from build123d import *

# Parameters (mm, degrees)
SKETCH1_W           = 137.287
SKETCH1_H           = 77.47
BOSS_EXTRUDE1_DEPTH = 17.78
SKETCH2_W           = 132.207
SKETCH2_H           = 67.31
CUT_EXTRUDE1_DEPTH  = 12.7
SKETCH4_R           = 11.43
CUT_EXTRUDE2_DEPTH  = 80.834956737
SKETCH5_W           = 137.287
SKETCH5_H           = 12.7
BOSS_EXTRUDE2_DEPTH = 1.27
SKETCH6_W           = 8.314266468
SKETCH6_H           = 19.05
CUT_EXTRUDE3_DEPTH  = 81.798878193
SKETCH9_W           = 137.287
SKETCH9_H           = 2
SKETCH9_W_2         = 10
SKETCH9_H_2         = 3
BOSS_EXTRUDE4_DEPTH = 3
SKETCH10_R          = 1.44
CUT_EXTRUDE4_DEPTH  = 84.591762855


with BuildPart() as part:
    # Sketch1 → Boss-Extrude1 (new body)
    with BuildSketch(Plane(origin=(0, 0, 0), x_dir=(1, 0, 0), z_dir=(0, 1, 0))):
        Rectangle(SKETCH1_W, SKETCH1_H)
    extrude(amount=BOSS_EXTRUDE1_DEPTH)

    # Sketch2 → Cut-Extrude1 (cut)
    with BuildSketch(Plane(origin=(0, 17.78, 0), x_dir=(1, 0, 0), z_dir=(0, 1, 0))):
        with Locations((2.54, 0)):
            Rectangle(SKETCH2_W, SKETCH2_H)
    extrude(amount=-CUT_EXTRUDE1_DEPTH, mode=Mode.SUBTRACT)

    # Sketch4 → Cut-Extrude2 (cut, through all)
    with BuildSketch(Plane(origin=(0, 5.08, 0), x_dir=(1, 0, 0), z_dir=(0, 1, 0))):
        with Locations(Location((43.7769, 0, 0), (0, 0, 270))):
            Circle(SKETCH4_R)
    extrude(amount=-CUT_EXTRUDE2_DEPTH, mode=Mode.SUBTRACT)

    # Sketch5 → Boss-Extrude2 (add)
    with BuildSketch(Plane(origin=(0, 17.78, 0), x_dir=(1, 0, 0), z_dir=(0, 1, 0))):
        with Locations((0, 32.385)):
            Rectangle(SKETCH5_W, SKETCH5_H)
        with Locations((0, -32.385)):
            Rectangle(SKETCH5_W, SKETCH5_H)
    extrude(amount=BOSS_EXTRUDE2_DEPTH)

    # Sketch6 → Cut-Extrude3 (cut, through all)
    with BuildSketch(Plane(origin=(0, 17.78, 0), x_dir=(1, 0, 0), z_dir=(0, 1, 0))):
        with Locations((-64.486366766, 0)):
            Rectangle(SKETCH6_W, SKETCH6_H)
    extrude(amount=-CUT_EXTRUDE3_DEPTH, mode=Mode.SUBTRACT)

    # Sketch9 → Boss-Extrude4 (add)
    with BuildSketch(Plane(origin=(0, 0, 0), x_dir=(-1, 0, 0), z_dir=(0, -1, 0))):
        with Locations((0, -39.735)):
            Rectangle(SKETCH9_W, SKETCH9_H)
        with Locations((0, 39.735)):
            Rectangle(SKETCH9_W, SKETCH9_H)
        with Locations((53.6435, -42.235)):
            Rectangle(SKETCH9_W_2, SKETCH9_H_2)
        with Locations((53.6435, 42.235)):
            Rectangle(SKETCH9_W_2, SKETCH9_H_2)
        with Locations((33.6435, -42.235)):
            Rectangle(SKETCH9_W_2, SKETCH9_H_2)
        with Locations((33.6435, 42.235)):
            Rectangle(SKETCH9_W_2, SKETCH9_H_2)
    extrude(amount=-BOSS_EXTRUDE4_DEPTH)

    # Sketch10 → Cut-Extrude4 (cut, through all)
    with BuildSketch(Plane(origin=(0, 0, 0), x_dir=(-1, 0, 0), z_dir=(0, -1, 0))):
        with Locations(Location((33.6435, -41.295, 0), (0, 0, 90))):
            Circle(SKETCH10_R)
        with Locations(Location((53.6435, -41.295, 0), (0, 0, 90))):
            Circle(SKETCH10_R)
        with Locations(Location((53.6435, 41.295, 0), (0, 0, 90))):
            Circle(SKETCH10_R)
        with Locations(Location((33.6435, 41.295, 0), (0, 0, 90))):
            Circle(SKETCH10_R)
    extrude(amount=-CUT_EXTRUDE4_DEPTH, mode=Mode.SUBTRACT)


solid = part.part
Source: CAD feature listing. Evaluate the final solid. Frame: model axes, mm. A direction names the side the tool comes from. Give positions to 0.01 mm unless a question says otherwise; leave off trailing zeros. Write each loop counter-clockwise with the first axis right and the second up, starting at its lowest first coordinate (ties: lowest second). Pieces come first, ordered by that corner, then holes. Notation, with made-up numbers: M -21.75,13 L 17.25,13 A7 cw 17.25,22 Z; hole C 29,82 d9. An arc over 180 degrees is marked long. Return JSON: item names as keys, results as strings. Group by question number.
1) Set-up query: faces 4 (the face through (-64, 1, -40.735)), 5 (the face through (21, 1, -40.735)), 6 (the face through (21, 1, 40.735)), 7 (the face through (-65, 9, 9.525)), 8 (the face through (-44, 1, 40.735)). Return all of +Z, -Z, +X, -X, +Y, -Y with unobstructed straight access to the full face (end or side cutting, diameter ignored); none if empty.
2) Pin query (flat end, axial travel): P1, Ø4, axis at y = 8.5, z = -25, coming from the +X side; P2, Ø1, axis at x = 39.5, y = 17, coming from the -Z side (3 decimals); P3, Ø5.5, axis at x = -66.5, z = 19, coming from the +Y side. Return the tip coordinate at first contact, or that it passes through.
3) Cut plane A-A, the plane z = 0. Output: boundary loops of the cut face in (x, y).
4) Pull-direction query (Y, two-part tool) for faces 1 (the face through (1, 3, -40)), 2 (the face through (-34, 1, 43.735)), 3 (the face through (-63.564, 12, -21)); classes: pulls with the +Y half, pulls with the -Y half, needs draft (parallel to the pull), parting line crosses it, or undercut.
5) Cut plane C-C, the plane x = 34.5. Output: boundary loops of the cut face in (y, z) (3 decimals).
6) Cut plane B-B, the plane y = 8. Output: boundary loops of the cut face in (x, z) (1 decimal).
7) Material intervals for line 1 along Y through (x, z) = (-20.5, -31); line 2 along Z through (x, y) = (-1, 13.5) (3 decimals); line 3 along Y through (x, z) = (15, -39.5), sorted ascending. Write a range as [from, to].
8) Cut plane D-D, the plane x = 10. Output: boundary loops of the cut face in (y, z) (3 decimals), plus the area to 3 significant figures.
Recorded:
{
 "1": {"face 4": "-Z, -X, +Y, -Y", "face 5": "-Z, +X, +Y, -Y", "face 6": "+Z, +X, +Y, -Y", "face 7": "-X, +Y, -Y", "face 8": "+Z, +Y, -Y"},
 "2": {"P1": "stops at x = -63.56", "P2": "stops at z = -38.735", "P3": "stops at y = 17.78"},
 "3": {"outline": "M -60.33,0 L 32.35,0 L 32.35,5.08 L -60.33,5.08 Z; M 55.21,0 L 68.64,0 L 68.64,5.08 L 55.21,5.08 Z"},
 "4": {"face 1": "pulls with the +Y half", "face 2": "needs draft", "face 3": "undercut"},
 "5": {"outline": "M 0,-40.735 L 3,-40.735 L 3,-38.735 L 19.05,-38.735 L 19.05,-26.035 L 17.78,-26.035 L 17.78,-33.655 L 5.08,-33.655 L 5.08,-6.677 L 0,-6.677 Z; M 0,6.677 L 5.08,6.677 L 5.08,33.655 L 17.78,33.655 L 17.78,26.035 L 19.05,26.035 L 19.05,38.735 L 3,38.735 L 3,40.735 L 0,40.735 Z"},
 "6": {"outline": "M -68.6,-38.7 L 68.6,-38.7 L 68.6,-33.7 L -63.6,-33.7 L -63.6,-9.5 L -68.6,-9.5 Z; M -68.6,9.5 L -63.6,9.5 L -63.6,33.7 L 68.6,33.7 L 68.6,38.7 L -68.6,38.7 Z"},
 "7": {"line 1": "y = [0, 5.08], [17.78, 19.05]", "line 2": "z = [-38.735, -33.655], [33.655, 38.735]", "line 3": "y = [0, 3]"},
 "8": {"outline": "M 0,-40.735 L 3,-40.735 L 3,-38.735 L 19.05,-38.735 L 19.05,-26.035 L 17.78,-26.035 L 17.78,-33.655 L 5.08,-33.655 L 5.08,33.655 L 17.78,33.655 L 17.78,26.035 L 19.05,26.035 L 19.05,38.735 L 3,38.735 L 3,40.735 L 0,40.735 Z", "area": "567 mm²"}
}
